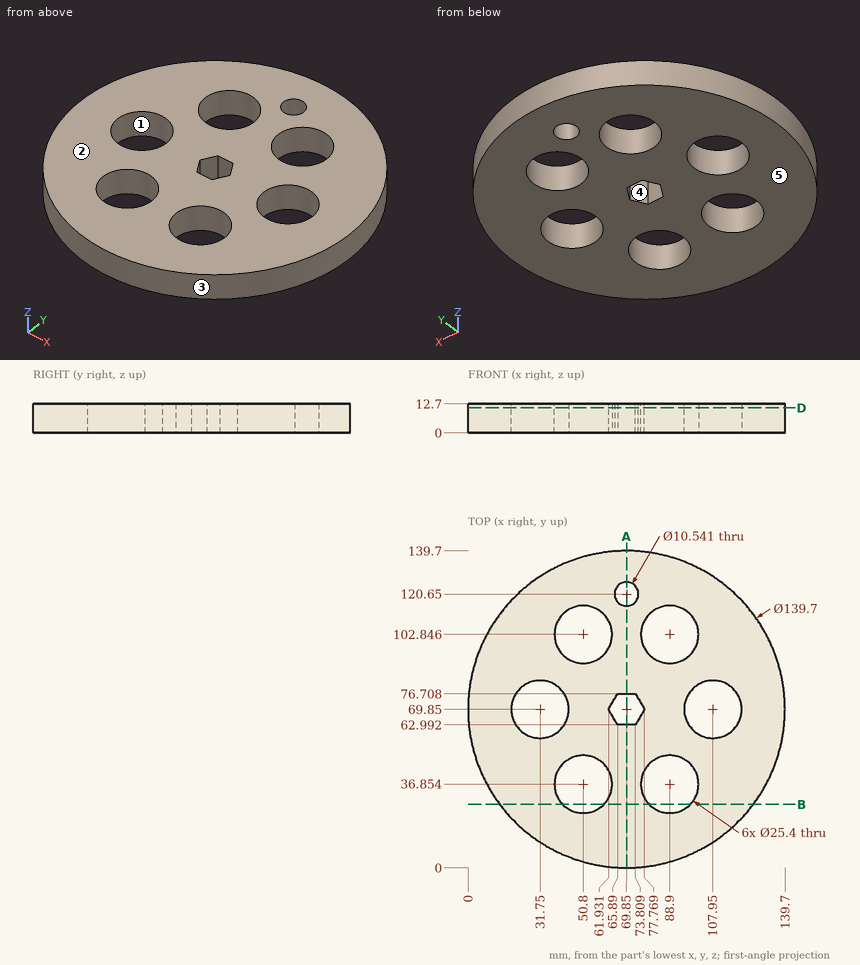
For this review, use the dimensioned drawing (mm, ordinates from the lowest corner) and the shaded views. A direction names the side the tool comes from. Coordinates: 2 decimals unless noted, no trailing zeros. Loops run counter-clockwise (first coordinate to the right, second up) from the corner with the lowest first, then second, coordinate; pieces in that order, holes last. Notation, with made-up numbers: (9.25, 22.5) -> (39.25, 22.5) arc R15 ccw to (39.25, 32.5) -> close; hole circle Ø10 at (58.5, 35.5). An arc over 180 degrees is marked (long way). Use a Markdown table: item, result. Add a question column.
Item 1: We need section D-D, the plane z = 11. Count the separate pieces of the cut face and the enclosed holes in it, and give its area (3 significant figures).
Item 2: Machinability: for the marked faces 4 and 5, which of the approach directions +Z, -Z, +X, -X, +Y, -Y give a long, thin tool a straight path to every point of the face, cutting with its end or side? Answer none if there is none.
Item 3: The part is to be moulded in two halves that separate along X. For the marked faces 1, 2 and 3, say which applies: +X half, -X half, draft (parallel to the pull), parting line (faces both ways), or undercut.
Item 4: We need section A-A, the plane x = 69.85. Write out the cut boundary in (y, z).
Item 5: Wall thickness on L1, parallel to Y at x = 69.85, z = 8; L2, parallel to Y at x = 50.8, z = 5.75 (1 decimal); L3, parallel to X at y = 80, z = 12.25 (1 decimal): over which ranges is each line inside the solid? List them lowest first. Write a range as from..to.
Item 6: We need section B-B, the plane y = 28. Write out the cut boundary in (x, z) (1 decimal).
Item 7: Clearance check with flat-ended pins moving along their axes: P1, Ø5, axis at x = 90, z = 11.5, coming from the +Y side; P2, Ø15, axis at x = 107.95, y = 69.85, coming from the +Z side; P3, Ø3, axis at y = 46.5, z = 4.5, coming from the -X side (1 decimal); P4, Ø2, axis at x = 122.5, z = 6, coming from the -Y side (1 decimal). State where each tip first meets the part, or that it passes through.
Numbers:
| question | item | result |
|---|---|---|
| 1 | separate pieces | 1 |
| 1 | enclosed holes | 8 |
| 1 | area | 12,000 mm^2 |
| 2 | face 4 | +Z, -Z |
| 2 | face 5 | -Z, +X, -X, +Y, -Y |
| 3 | face 1 | undercut |
| 3 | face 2 | draft |
| 3 | face 3 | parting line |
| 4 | outline | (0, 0) -> (62.99, 0) -> (62.99, 12.7) -> (0, 12.7) -> close; (76.71, 0) -> (115.38, 0) -> (115.38, 12.7) -> (76.71, 12.7) -> close; (125.92, 0) -> (139.7, 0) -> (139.7, 12.7) -> (125.92, 12.7) -> close |
| 5 | L1 | y = 0..62.99, 76.71..115.38, 125.92..139.7 |
| 5 | L2 | y = 2.6..24.2, 49.6..90.1, 115.5..137.1 |
| 5 | L3 | x = 0.7..24.1, 39.4..100.3, 115.6..139 |
| 6 | outline | (13.9, 0) -> (41.7, 0) -> (41.7, 12.7) -> (13.9, 12.7) -> close; (59.9, 0) -> (79.8, 0) -> (79.8, 12.7) -> (59.9, 12.7) -> close; (98, 0) -> (125.8, 0) -> (125.8, 12.7) -> (98, 12.7) -> close |
| 7 | P1 | stops at y = 137.43 |
| 7 | P2 | passes through |
| 7 | P3 | stops at x = 3.5 |
| 7 | P4 | stops at y = 22.8 |
